Geometry: final body of the model. Coordinates: model frame, mm. Face numbers are marked on the shaded views. A direction names the side the tool comes from. Give positions to 0.01 mm unless a question says otherwise; leave off trailing zeros. Loops run counter-clockwise (first coordinate to the right, second up) from the corner with the lowest first, then second, coordinate; pieces in that order, holes last. Notation, with made-up numbers: (4, 78.25) - (47, 78.25) arc R22 cw to (47, 112.25) - close; hole circle Ø8 at (52.5, -13.75). An arc over 180 degrees is marked (long way). Use one line per item in the form item = value.
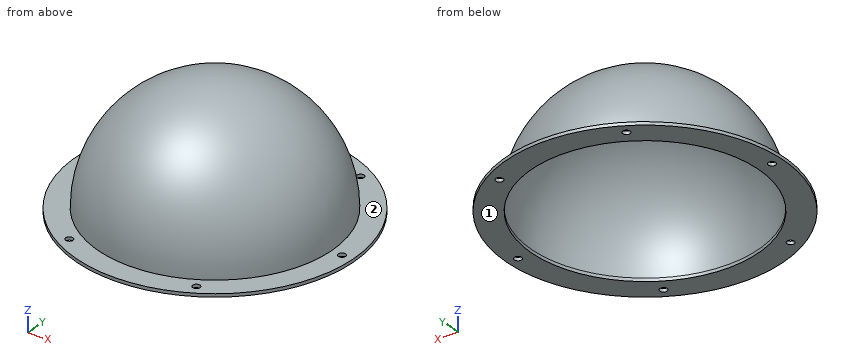
```python
from build123d import *

# Parameters (mm, degrees)
SKETCH2_R          = 3.175
CUT_EXTRUDE1_DEPTH = 199.583496293
CIRPATTERN1_COUNT  = 6


with BuildPart() as part:
    # Sketch1 → Revolve1 (revolve)
    with BuildSketch(Plane(origin=(0, 0, 0), x_dir=(1, 0, 0), z_dir=(0, 1, 0))):
        with BuildLine():
            Line((98.821875, 0), (98.821875, 2.778125))
            Line((98.821875, 2.778125), (120.65, 2.778125))
            Line((120.65, 2.778125), (120.65, 0))
            Line((120.65, 0), (101.6, 0))
            ThreePointArc((101.6, 0), (71.842048969, -71.842048969), (0, -101.6))
            Line((0, -101.6), (0, -98.821875))
            ThreePointArc((0, -98.821875), (69.877617942, -69.877617942), (98.821875, 0))
        make_face()
    revolve(axis=Axis((0, 0, 0), (0, 0, 1)))

    # Sketch2 → Cut-Extrude1 (cut, symmetric)
    with BuildSketch(Plane.XY):
        with Locations((111.125, 0)):
            Circle(SKETCH2_R)
    cut_extrude1 = extrude(amount=CUT_EXTRUDE1_DEPTH, both=True, mode=Mode.SUBTRACT)

    # CirPattern1: Cut-Extrude1 ×6 about axis
    cirpattern1_axis = Axis((0, 0, 0), (0, 0, 1))
    for i in range(1, CIRPATTERN1_COUNT):
        add(cut_extrude1.rotate(cirpattern1_axis, i * 360 / CIRPATTERN1_COUNT), mode=Mode.SUBTRACT)


solid = part.part
```
(1) Cut plane A-A (y = 0). Return the cut outline in (x, z), plus the area to 3 significant figures.
Solution:
outline = (-120.65, -2.78) - (-114.3, -2.78) - (-114.3, 0) - (-120.65, 0) - close; (-107.95, -2.78) - (-98.82, -2.78) - (-98.82, 0) arc R98.82 cw to (98.82, 0) - (98.82, -2.78) - (107.95, -2.78) - (107.95, 0) - (101.6, 0) arc R101.6 ccw to (-101.6, 0) - (-107.95, 0) - close; (114.3, -2.78) - (120.65, -2.78) - (120.65, 0) - (114.3, 0) - close
area = 961 mm2
(2) Cut plane B-B (x = 68). Return the cut outline in (y, z), plus the area to 3 significant figures.
Solution:
outline = (-99.66, -2.78) - (-71.71, -2.78) - (-71.71, 0) arc R71.71 cw to (71.71, 0) - (71.71, -2.78) - (99.66, -2.78) - (99.66, 0) - (75.49, 0) arc R75.49 ccw to (-75.49, 0) - (-99.66, 0) - close
area = 1,030 mm2
(3) Cut plane D-D (x = 0). Return the cut outline in (y, z), plus the area to 3 significant figures.
Solution:
outline = (-120.65, -2.78) - (-98.82, -2.78) - (-98.82, 0) arc R98.82 cw to (98.82, 0) - (98.82, -2.78) - (120.65, -2.78) - (120.65, 0) - (101.6, 0) arc R101.6 ccw to (-101.6, 0) - (-120.65, 0) - close
area = 996 mm2
(4) Material intervals for L1, parallel to Y at x = 0, z = -1.1; L2, parallel to Z at x = -55.5, y = -85.5; L3, parallel to X at y = 76, z = 9.5, sorted ascending. Write a range as from..to.
Solution:
L1 = -120.65..-98.82, 98.82..120.65
L2 = -2.78..0
L3 = -66.76..-62.45, 62.45..66.76
(5) Pin query (flat end, axial travel): P1, Ø10, axis at x = -43, z = 46, coming from the -Y side; P2, Ø5, axis at x = 111.125, y = 0, coming from the +Z side; P3, Ø1.5, axis at y = -59, z = 70, coming from the -X side; P4, Ø4, axis at y = 31, z = 84.5, coming from the +X side. Return the tip coordinate at first contact, or that it passes through.
Solution:
P1 = -83.44
P2 = through
P3 = -45.59
P4 = 50.77
(6) Access query for the marked faces 1 and 2. Directions: +Z, -Z, +X, -X, +Y, -Y. A direction counts if a zero-diameter tool reaches every point of the face in a straight line with its end or side. Return the directions, or none.
Solution:
face_1 = -Z, +X, -X, +Y, -Y
face_2 = +Z
(7) Cut plane C-C (z = 36). Return the cut outline in (x, y).
Solution:
outline = circle Ø190.02 at (0, 0); hole circle Ø184.06 at (0, 0)
